from build123d import *

# Parameters (mm, degrees)
SKETCH_1_W            = 1.320722759
SKETCH_1_H            = 1.348576416
EXTRUDE_2_DEPTH       = 2.06
SKETCH_1_3_W          = 2.567505851
SKETCH_1_3_H          = 1.451984885
EXTRUDE_3_DEPTH       = 1.72
SKETCH_1_4_W          = 10.768406503
SKETCH_1_4_H          = 12.814051925
EXTRUDE_4_DEPTH       = 2.94
SKETCH_1_5_W          = 1.751728556
SKETCH_1_5_H          = 3.911393899
EXTRUDE_5_DEPTH       = 1.66
SKETCH_1_6_W          = 2.863837954
SKETCH_1_6_H          = 3.684536573
EXTRUDE_6_DEPTH       = 2.23
SKETCH_1_7_W          = 0.666899611
SKETCH_1_7_H          = 1.198197092
EXTRUDE_7_DEPTH       = 1.64
SKETCH_1_8_W          = 1.201543901
SKETCH_1_8_H          = 1.909822412
EXTRUDE_8_DEPTH       = 1.7
EXTRUDE_9_DEPTH       = 1.2
EXTRUDE_10_DEPTH      = 1.45
EXTRUDE_10_DEPTH_BACK = 6.1


with BuildPart() as part:
    # Sketch 1 → Extrude 2 (new body)
    with BuildSketch(Plane(origin=(0, 0, 0), x_dir=(1, 0, 0), z_dir=(0, 1, 0))):
        with Locations((2.886090317, 14.593344496)):
            Rectangle(SKETCH_1_W, SKETCH_1_H)
    extrude(amount=EXTRUDE_2_DEPTH)



with BuildPart() as body_2:
    # Sketch 1_3 → Extrude 3 (new body)
    with BuildSketch(Plane(origin=(0, 0, 0), x_dir=(1, 0, 0), z_dir=(0, 1, 0))):
        with Locations((1.758272699, 3.179573222)):
            Rectangle(SKETCH_1_3_W, SKETCH_1_3_H)
    extrude(amount=EXTRUDE_3_DEPTH)


with BuildPart() as body_3:
    # Sketch 1_4 → Extrude 4 (new body)
    with BuildSketch(Plane(origin=(0, 0, 0), x_dir=(1, 0, 0), z_dir=(0, 1, 0))):
        with Locations((12.311476922, 8.860606741)):
            Rectangle(SKETCH_1_4_W, SKETCH_1_4_H)
    extrude(amount=EXTRUDE_4_DEPTH)


with BuildPart() as body_4:
    # Sketch 1_5 → Extrude 5 (new body)
    with BuildSketch(Plane(origin=(0, 0, 0), x_dir=(1, 0, 0), z_dir=(0, 1, 0))):
        with Locations((19.907360624, 7.039973628)):
            Rectangle(SKETCH_1_5_W, SKETCH_1_5_H)
    extrude(amount=EXTRUDE_5_DEPTH)


with BuildPart() as body_5:
    # Sketch 1_6 → Extrude 6 (new body)
    with BuildSketch(Plane(origin=(0, 0, 0), x_dir=(1, 0, 0), z_dir=(0, 1, 0))):
        with Locations((19.351305925, 13.425364418)):
            Rectangle(SKETCH_1_6_W, SKETCH_1_6_H)
    extrude(amount=EXTRUDE_6_DEPTH)


with BuildPart() as body_6:
    # Sketch 1_7 → Extrude 7 (new body)
    with BuildSketch(Plane(origin=(0, 0, 0), x_dir=(1, 0, 0), z_dir=(0, 1, 0))):
        with Locations((0.617323995, 14.668534158)):
            Rectangle(SKETCH_1_7_W, SKETCH_1_7_H)
    extrude(amount=EXTRUDE_7_DEPTH)


with BuildPart() as body_7:
    # Sketch 1_8 → Extrude 8 (new body)
    with BuildSketch(Plane(origin=(0, 0, 0), x_dir=(1, 0, 0), z_dir=(0, 1, 0))):
        with Locations((20.00563527, 3.683898)):
            Rectangle(SKETCH_1_8_W, SKETCH_1_8_H)
    extrude(amount=EXTRUDE_8_DEPTH)


with BuildPart() as part_1:
    add(part.part)

    add(body_2.part)  # Extrude 9 merges body 2

    add(body_3.part)  # Extrude 9 merges body 3

    add(body_4.part)  # Extrude 9 merges body 4

    add(body_5.part)  # Extrude 9 merges body 5

    add(body_6.part)  # Extrude 9 merges body 6

    add(body_7.part)  # Extrude 9 merges body 7
    # Sketch 1_9 → Extrude 9 (add)
    with BuildSketch(Plane(origin=(0, 0, 0), x_dir=(1, 0, 0), z_dir=(0, 1, 0))):
        with BuildLine():
            Line((2, 0), (19.15, 0))
            ThreePointArc((19.15, 0), (20.564213562, 0.585786438), (21.15, 2))
            Line((21.15, 2), (21.15, 15.77))
            ThreePointArc((21.15, 15.77), (20.564213562, 17.184213562), (19.15, 17.77))
            Line((19.15, 17.77), (2, 17.77))
            ThreePointArc((2, 17.77), (0.585786438, 17.184213562), (0, 15.77))
            Line((0, 15.77), (0, 2))
            ThreePointArc((0, 2), (0.585786438, 0.585786438), (2, 0))
        make_face()
    extrude(amount=EXTRUDE_9_DEPTH)

    # Sketch 4 → Extrude 10 (add, two sides: drawn at the far end of the back side and taken through both)
    with BuildSketch(Plane.ZY.offset(-EXTRUDE_10_DEPTH_BACK)):
        with BuildLine():
            Line((-12.37, 1.2), (-5.41, 1.2))
            ThreePointArc((-5.41, 1.2), (-4.702893219, 1.492893219), (-4.41, 2.2))
            Line((-4.41, 2.2), (-4.41, 3.46))
            ThreePointArc((-4.41, 3.46), (-4.702893219, 4.167106781), (-5.41, 4.46))
            Line((-5.41, 4.46), (-12.37, 4.46))
            ThreePointArc((-12.37, 4.46), (-13.077106781, 4.167106781), (-13.37, 3.46))
            Line((-13.37, 3.46), (-13.37, 2.2))
            ThreePointArc((-13.37, 2.2), (-13.077106781, 1.492893219), (-12.37, 1.2))
        make_face()
    extrude(amount=EXTRUDE_10_DEPTH + EXTRUDE_10_DEPTH_BACK)


solid = part_1.part
Verification items for the finished model (mm, model axes). A direction names the side the tool comes from. Coordinates: 2 decimals unless noted, no trailing zeros. Order: outer loops, then holes, each group sorted by start corner. A loop starts at its lowest first (then second) coordinate and runs counter-clockwise, first axis right, second up. Notation, with made-up numbers: M 76.25,20.25 L 119.25,20.25 A14 cw 119.25,28.25 Z; hole C 73,3.5 d5. An arc over 180 degrees is marked long. Write each question's results on one line, items separated by ' | '.
1) Access from +Z, -Z, +X, -X, +Y, -Y to the whole of each face (thin tool, end or side, straight path). Record for faces 1 (the face through (19, 2.23, -13)), 2 (the face through (6, 1.2, -13)), 3 (the face through (2, 3, -4.41)).
Solved:
face 1: +Z, -Z, +X, +Y | face 2: none | face 3: +Z, -X, +Y
2) Section check C-C on x = 13. Record the cut outline in (y, z), plus the area to 3 significant figures.
Solved:
outline: M 0,-17.77 L 1.2,-17.77 L 1.2,-15.27 L 2.94,-15.27 L 2.94,-2.45 L 1.2,-2.45 L 1.2,0 L 0,0 Z | area: 43.6 mm²
3) Section check A-A on y = 2.55. Record the cut outline in (x, z), plus the area to 3 significant figures.
Solved:
outline: M -1.45,-13.37 L 6.1,-13.37 L 6.1,-4.41 L -1.45,-4.41 Z; M 6.93,-15.27 L 17.7,-15.27 L 17.7,-2.45 L 6.93,-2.45 Z | area: 206 mm²
4) Section check D-D on y = 0.85. Record the cut outline in (x, z).
Solved:
outline: M 0,-15.77 A2 ccw 2,-17.77 L 19.15,-17.77 A2 ccw 21.15,-15.77 L 21.15,-2 A2 ccw 19.15,0 L 2,0 A2 ccw 0,-2 Z
5) Section check B-B on z = -6. Record the cut outline in (x, y), plus the area to 3 significant figures.
Solved:
outline: M -1.45,1.2 L 0,1.2 L 0,0 L 21.15,0 L 21.15,1.2 L 20.78,1.2 L 20.78,1.66 L 19.03,1.66 L 19.03,1.2 L 17.7,1.2 L 17.7,2.94 L 6.93,2.94 L 6.93,1.2 L 6.1,1.2 L 6.1,4.46 L -1.45,4.46 Z | area: 69.5 mm²
6) Scan lines: line 1 along Y through (x, z) = (13.5, -5.5); line 2 along X through (y, z) = (0.2, -4.5); line 3 along Z through (x, y) = (1.75, 2.4). Record each from-to range of solid material in increasing order. Write a range as [from, to].
Solved:
line 1: y = [0, 2.94] | line 2: x = [0, 21.15] | line 3: z = [-13.37, -4.41]
7) Gauge pin test, flat ends, axial feed: pin 1 Ø1 at (x, z) = (20, -4) entering from +Y; pin 2 Ø1.6 at (y, z) = (2.5, -8) entering from +X; pin 3 Ø2 at (x, z) = (5, -3) entering from +Y; pin 4 Ø0.8 at (x, y) = (19, 1.5) entering from +Z. Record the tip position at first contact, or that the pin passes through.
Solved:
pin 1: stops at y = 1.7 | pin 2: stops at x = 17.7 | pin 3: stops at y = 1.2 | pin 4: stops at z = 0
8) Release check for a two-part mould opening along X. For faces 4 (the face through (6.927, 2, -9)), 5 (the face through (20.783, 2, -13)), 6 (the face through (-1.45, 3, -9)), 7 (the face through (3, 2.06, -15)) record: pulls with the +X half, pulls with the -X half, needs draft (parallel to the pull), parting line crosses it, or undercut.
Solved:
face 4: undercut | face 5: pulls with the +X half | face 6: pulls with the -X half | face 7: needs draft
